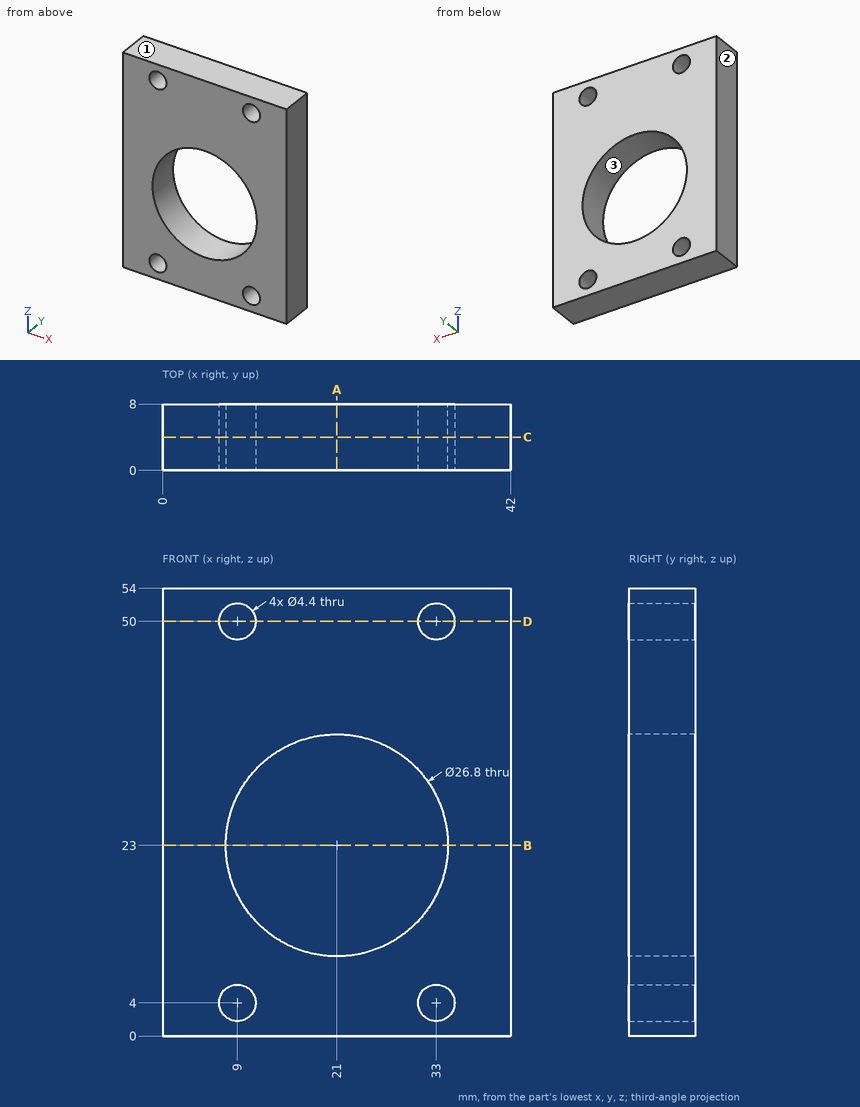
The drawing under review shows one solid part. Ordinate dimensions are in mm from its lowest x, y, z. Round coordinates to 2 decimals unless told otherwise and drop trailing zeros. Order: outer loops, then holes, each group sorted by start corner. A loop starts at its lowest first (then second) coordinate and runs counter-clockwise, first axis right, second up. Notation, with made-up numbers: M -39,43 L 5,43 A10 cw 5,61 Z; hole C 46.5,37.5 d5. An arc over 180 degrees is marked long. Answer as CSV lines item,"result". Start each with the question number.
1) Add section A-A (x = 21). Give the boundary of the cut face in (y, z), then the cut area to 3 significant figures.
2) Add section C-C (y = 4). Give the boundary of the cut face in (x, z).
3) Add section B-B (z = 23). Give the boundary of the cut face in (x, y).
4) The part is to be moulded in two halves that separate along X. For the marked faces 1, 2 and 3, say which applies: +X half, -X half, draft (parallel to the pull), parting line (faces both ways), or undercut.
5) For pin 1 Ø6 at (x, z) = (27, 6) entering from -Y, flat-tipped, find the tip position at first contact; note if it passes through.
6) Add section D-D (z = 50). Give the boundary of the cut face in (x, y), then the cut area to 3 significant figures.
7) Wall thickness on line 1 along X through (y, z) = (6.25, 50); line 2 along Z through (x, y) = (33, 5.5); line 3 along Z through (x, y) = (31, 6.25): over which ranges is each line inside the solid? List them lowest first. Write a range as [from, to].
Resolved:
1,outline,"M 0,0 L 8,0 L 8,9.6 L 0,9.6 Z; M 0,36.4 L 8,36.4 L 8,54 L 0,54 Z"
1,area,"218 mm^2"
2,outline,"M 0,0 L 42,0 L 42,54 L 0,54 Z; hole C 9,4 d4.4; hole C 9,50 d4.4; hole C 21,23 d26.8; hole C 33,4 d4.4; hole C 33,50 d4.4"
3,outline,"M 0,0 L 7.6,0 L 7.6,8 L 0,8 Z; M 34.4,0 L 42,0 L 42,8 L 34.4,8 Z"
4,face 1,"draft"
4,face 2,"-X half"
4,face 3,"undercut"
5,pin 1,"y = 0"
6,outline,"M 0,0 L 6.8,0 L 6.8,8 L 0,8 Z; M 11.2,0 L 30.8,0 L 30.8,8 L 11.2,8 Z; M 35.2,0 L 42,0 L 42,8 L 35.2,8 Z"
6,area,"266 mm^2"
7,line 1,"[0, 6.8], [11.2, 30.8], [35.2, 42]"
7,line 2,"[0, 1.8], [6.2, 17.04], [28.96, 47.8], [52.2, 54]"
7,line 3,"[0, 3.08], [4.92, 14.08], [31.92, 49.08], [50.92, 54]"
